from build123d import *

# Parameters (mm, degrees)
BOSS_EXTRUDE1_DEPTH = 20


with BuildPart() as part:
    # Sketch1 → Boss-Extrude1 (new body)
    with BuildSketch(Plane.XY):
        Polygon((0, 0), (303.108891325, 0), (303.108891325, 175), align=None)
        Polygon((283.108891325, 140.358983849), (74.641016151, 20), (283.108891325, 20), align=None, mode=Mode.SUBTRACT)
    extrude(amount=BOSS_EXTRUDE1_DEPTH)


solid = part.part
Input: part model. Units: mm. Frame: model coordinates. A direction names the side the tool comes from. Coordinates: 2 decimals unless noted, no trailing zeros. Loops run counter-clockwise (first coordinate to the right, second up) from the corner with the lowest first, then second, coordinate; pieces in that order, holes last. Notation, with made-up numbers: (-32, -33.5) -> (3, -33.5) arc R16 ccw to (3, -16.5) -> close; hole circle Ø11 at (42.5, 60.5). An arc over 180 degrees is marked (long way). Write item = value, one per line. Start each with the question number.
Item 1: First-contact query: P1, Ø12, axis at x = 44.5, z = 10, coming from the -Y side; P2, Ø12, axis at x = 100.5, z = 13, coming from the +Y side; P3, Ø12, axis at y = 72, z = 7, coming from the -X side; P4, Ø10, axis at y = 115, z = 16, coming from the -X side. Flat tips, straight axial feed; report the tip coordinate or a pass-through.
Item 2: Cut plane A-A, the plane x = 255. Return loops of the section in (y, z).
Item 3: Mould query, pull axis X, two halves, no side actions, for faces 3 (the face through (185, 88, 0)), 4 (the face through (303.109, 86, 10)), 5 (the face through (177, 20, 10)), 6 (the face through (180.3, 81, 9.9)). Classes: pulls with the +X half, pulls with the -X half, needs draft (parallel to the pull), parting line crosses it, or undercut.
Item 4: Material intervals for line 1 (Y direction, x = 256.5, z = 8.25); line 2 (Y direction, x = 202, z = 9.5); line 3 (X direction, y = 36, z = 6.5), sorted ascending.
Item 5: Cut plane D-D, the plane y = 15.5. Return loops of the section in (x, z).
Item 6: Reachability of faces 1 (the face through (283.109, 79, 10)), 2 (the face through (153.676, 88.725, 9.86)) from +Z, -Z, +X, -X, +Y, -Y: full face, straight path, thin tool, end or side. Return the list, or none.
Item 7: Cut plane B-B, the plane y = 71.5. Return loops of the section in (x, z), plus the area to 3 significant figures.
Item 8: Cut plane C-C, the plane z = 5.25. Return loops of the section in (x, y), plus the area to 3 significant figures.
Ans:
q1.P1 = 0
q1.P2 = 61.49
q1.P3 = 114.32
q1.P4 = 190.53
q2.outline = (0, 0) -> (20, 0) -> (20, 20) -> (0, 20) -> close; (124.13, 0) -> (147.22, 0) -> (147.22, 20) -> (124.13, 20) -> close
q3.face_3 = needs draft
q3.face_4 = pulls with the +X half
q3.face_5 = undercut
q3.face_6 = undercut
q4.line_1 = 0 to 20, 125 to 148.09
q4.line_2 = 0 to 20, 93.53 to 116.62
q4.line_3 = 62.35 to 102.35, 283.11 to 303.11
q5.outline = (26.85, 0) -> (303.11, 0) -> (303.11, 20) -> (26.85, 20) -> close
q6.face_1 = +Z, -Z
q6.face_2 = +Z, -Z, -X, +Y
q7.outline = (123.84, 0) -> (163.84, 0) -> (163.84, 20) -> (123.84, 20) -> close; (283.11, 0) -> (303.11, 0) -> (303.11, 20) -> (283.11, 20) -> close
q7.area = 1,200 mm²
q8.outline = (0, 0) -> (303.11, 0) -> (303.11, 175) -> close; hole (74.64, 20) -> (283.11, 20) -> (283.11, 140.36) -> close
q8.area = 14,000 mm²
